Design review of the part built by this model. Coordinates are the model's own, in mm. A direction names the side the tool comes from. Round coordinates to 2 decimals unless told otherwise and drop trailing zeros. Order: outer loops, then holes, each group sorted by start corner. A loop starts at its lowest first (then second) coordinate and runs counter-clockwise, first axis right, second up. Notation, with made-up numbers: (69, 40) - (91, 40) arc R17 ccw to (91, 49) - close; hole circle Ø2 at (9.5, 25.25). An arc over 180 degrees is marked (long way). Write item = value, one per line.
from build123d import *

# Parameters (mm, degrees)
SKETCH039_R   = 3
SKETCH039_R_2 = 1.75
SKETCH039_W   = 3.25
SKETCH039_H   = 2.2
PAD022_DEPTH  = 2.5
SKETCH026_W   = 10
SKETCH026_H   = 9
PAD020_DEPTH  = 2
PAD019_DEPTH  = 5.5
FILLET003_R   = 1.3
FILLET004_R   = 0.99


with BuildPart() as pad_button_zoom_holes:
    # Sketch039 → Pad022 (new body)
    with BuildSketch(Plane.XY):
        Circle(SKETCH039_R)
        Circle(SKETCH039_R_2, mode=Mode.SUBTRACT)
        with Locations((-7.5, 0)):
            Rectangle(SKETCH039_W, SKETCH039_H)
        with Locations((7.5, 0)):
            Rectangle(SKETCH039_W, SKETCH039_H)
    extrude(amount=PAD022_DEPTH)


with BuildPart() as pad_button_zoom_cutout:
    # Sketch026 → Pad020 (new body)
    with BuildSketch(Plane.XY.offset(4.5)):
        Rectangle(SKETCH026_W, SKETCH026_H)
    extrude(amount=PAD020_DEPTH)


with BuildPart() as cut_button_zoom_final:
    # Sketch025 → Pad019 (new body)
    with BuildSketch(Plane.XY):
        with BuildLine():
            ThreePointArc((11.557852, 3.5), (0, 3.566794), (-11.557852, 3.5))
            ThreePointArc((-11.557852, 3.5), (-12.578424, 3.066971), (-12.999999, 2.041615))
            ThreePointArc((-12.999999, 2.041615), (-13.000368, 0), (-13, -2.041615))
            ThreePointArc((-13, -2.041615), (-12.578425, -3.066972), (-11.557852, -3.5))
            ThreePointArc((-11.557852, -3.5), (0, -3.566794), (11.557852, -3.5))
            ThreePointArc((11.557852, -3.5), (12.578425, -3.066972), (13, -2.041615))
            ThreePointArc((13, -2.041615), (13.000368, 0), (12.999999, 2.041615))
            ThreePointArc((12.999999, 2.041615), (12.578424, 3.066971), (11.557852, 3.5))
        make_face()
    extrude(amount=PAD019_DEPTH)

    # Cut007: cut Pad (button zoom cutout)
    add(pad_button_zoom_cutout.part, mode=Mode.SUBTRACT)

    # Fillet003
    fillet003_edges = [cut_button_zoom_final.edges().sort_by_distance(p)[0] for p in [
        (-5, 3.554294, 5),
        (5, 3.554294, 5),
        (-5, -3.554294, 5),
        (5, -3.554294, 5),
    ]]
    fillet(fillet003_edges, radius=FILLET003_R)

    # Fillet004
    fillet004_edges = [cut_button_zoom_final.edges().sort_by_distance(p)[0] for p in [
        (-8.933057, 3.526894, 5.5),
        (8.933057, 3.526894, 5.5),
        (-5.383665, 3.169057, 5.5),
        (-12.578424, 3.066971, 5.5),
        (-5, 0, 5.5),
        (-13.000368, 0, 5.5),
        (-5.383665, -3.169057, 5.5),
        (-12.578425, -3.066972, 5.5),
        (-8.933057, -3.526894, 5.5),
        (12.578424, 3.066971, 5.5),
        (5.383665, 3.169057, 5.5),
        (5, 0, 5.5),
        (13.000368, 0, 5.5),
        (5.383665, -3.169057, 5.5),
        (12.578425, -3.066972, 5.5),
        (8.933057, -3.526894, 5.5),
    ]]
    fillet(fillet004_edges, radius=FILLET004_R)

    # Cut: cut Pad (button zoom holes)
    add(pad_button_zoom_holes.part, mode=Mode.SUBTRACT)


solid = cut_button_zoom_final.part
1) For faces 4 (the cylindrical face through (-5.28, 0.03, 5.2)), 5 (the flat face through (0, -2, 2.5)), 6 (the cylindrical face through (0.162, 3.567, 2.223)), list the 3-axis set-ups (+Z, -Z, +X, -X, +Y, -Y) from which the entire face can be reached by the end or side of a thin tool; tool diameter is ignored.
Findings:
face_4 = +Z, +Y, -Y
face_5 = -Z
face_6 = +Z, -Z, +Y
2) We need section B-B on x = 0. Write out the cut boundary in (y, z), and give its area (3 significant figures).
Findings:
outline = (-3.57, 0) - (-3, 0) - (-3, 2.5) - (-1.75, 2.5) - (-1.75, 0) - (1.75, 0) - (1.75, 2.5) - (3, 2.5) - (3, 0) - (3.57, 0) - (3.57, 4.5) - (-3.57, 4.5) - close
area = 25.9 mm^2
3) Clearance check with flat-ended pins moving along their axes: pin 1 Ø1 at (x, z) = (-4.5, 2.5) entering from +Y; pin 2 Ø3.5 at (x, y) = (-1, 0.5) entering from +Z; pin 3 Ø1.2 at (x, z) = (7.5, 1) entering from -Y; pin 4 Ø1 at (x, y) = (0.5, 0.5) entering from -Z. State where each tip first meets the part, or that it passes through.
Findings:
pin_1 = 3.56
pin_2 = 4.5
pin_3 = -3.54
pin_4 = 0
4) To check wall thickness, follow L1, parallel to Y at x = 0, z = 0.95; L2, parallel to X at y = 0.75, z = 0.45 (3 decimals); L3, parallel to X at y = 0, z = 4.6. State the ranges of each line that lie inside material, in increasing order. Write a range as from..to.
Findings:
L1 = -3.57..-3, -1.75..1.75, 3..3.57
L2 = -13..-9.125, -5.875..-2.905, -1.581..1.581, 2.905..5.875, 9.125..13
L3 = -13..-5, 5..13
5) We need section C-C on z = 3.6. Write out the cut boundary in (x, y), and give its area (3 significant figures).
Findings:
outline = (-13, -2.04) arc R1.46 ccw to (-11.56, -3.5) arc R1000 ccw to (11.56, -3.5) arc R1.46 ccw to (13, -2.04) arc R5655.62 ccw to (13, 2.04) arc R1.46 ccw to (11.56, 3.5) arc R1000 ccw to (-11.56, 3.5) arc R1.46 ccw to (-13, 2.04) arc R5655.62 ccw to start
area = 182 mm^2
6) We need section A-A on z = 2.2. Write out the cut boundary in (x, y) (3 decimals).
Findings:
outline = (-13, -2.042) arc R1.459 ccw to (-11.558, -3.5) arc R1000.003 ccw to (11.558, -3.5) arc R1.459 ccw to (13, -2.042) arc R5655.62 ccw to (13, 2.042) arc R1.459 ccw to (11.558, 3.5) arc R1000.003 ccw to (-11.558, 3.5) arc R1.459 ccw to (-13, 2.042) arc R5655.62 ccw to start; circle Ø3.5 at (0, 0); hole (-9.125, -1.1) - (-5.875, -1.1) - (-5.875, 1.1) - (-9.125, 1.1) - close; hole circle Ø6 at (0, 0); hole (5.875, -1.1) - (9.125, -1.1) - (9.125, 1.1) - (5.875, 1.1) - close
7) The part is to be moulded in two halves that separate along Y. For faces 1 (the flat face through (9, 0, 5.5)), 2 (the flat face through (7, 1.1, 1)), 3 (the cylindrical face through (-0.162, -3.567, 2.223)), say which applies: released by +Y, released by -Y, zero draft, split by the parting line, or undercut.
Findings:
face_1 = zero draft
face_2 = undercut
face_3 = released by -Y
8) We need section D-D on x = -3.5. Write out the cut boundary in (y, z), and give its area (3 significant figures).
Findings:
outline = (-3.56, 0) - (3.56, 0) - (3.56, 4.5) - (-3.56, 4.5) - close
area = 32.0 mm^2
